Geometry: final body of the model. Coordinates: model frame, mm. A direction names the side the tool comes from. Give positions to 0.01 mm unless a question says otherwise; leave off trailing zeros. Loops run counter-clockwise (first coordinate to the right, second up) from the corner with the lowest first, then second, coordinate; pieces in that order, holes last. Notation, with made-up numbers: (-7.5, -10) -> (-2.5, -10) arc R13 ccw to (-2.5, 1) -> close; hole circle Ø5 at (1.5, -32.75). An arc over 180 degrees is marked (long way). One line per question, with ' | ' between items. Start each with the question number.
Item 1: Mould query, pull axis Z, two halves, no side actions, for faces 3 (the cylindrical face through (-1.521, 5.406, -5.712)), 4 (the cylindrical face through (-1.479, 19.248, -0.713)), 5 (the flat face through (0, 10, -11)). Classes: released by +Z, released by -Z, zero draft, split by the parting line, or undercut.
Item 2: Pin query (flat end, axial travel): P1, Ø9, axis at x = 9, z = -0.5, coming from the +Y side; P2, Ø9.5, axis at x = 12.5, y = 7, coming from the -Z side; P3, Ø3.5, axis at y = 15, z = -7, coming from the +X side. Return the tip coordinate at first contact, or that it passes through.
Item 3: Set-up query: faces 1 (the flat face through (-2, 20, -10)), 2 (the flat face through (11, 7, 0)). Return all of +Z, -Z, +X, -X, +Y, -Y with unobstructed straight access to the full face (end or side cutting, diameter ignored); none if empty.
Item 4: Section B-B on z = -7. Return loops of the section in (x, y).
Item 5: Section A-A on y = 5. Return loops of the section in (x, z).
Item 6: Section C-C on z = -10.75. Return loops of the section in (x, y).
Item 7: Material intervals for line 1 along Y through (x, z) = (-1, -7); line 2 along X through (y, z) = (9.5, -5.25); line 3 along Z through (x, y) = (7, 13.5), sorted ascending. Write a range as [from, to].
Item 8: Section D-D on x = 10. Return loops of the section in (y, z), then the cut area to 3 significant figures.
from build123d import *

# Parameters (mm, degrees)
BOSS_EXTRUDE1_DEPTH            = 20
F_2_7_2_7_DIAMETER_HOLE1_D     = 2.7
F_2_7_2_7_DIAMETER_HOLE1_DEPTH = 15
F_2_7_2_7_DIAMETER_HOLE1_TIP   = 0.811161836
SKETCH4_W                      = 20
SKETCH4_H                      = 3
CUT_EXTRUDE1_DEPTH             = 5
FILLET2_R                      = 2.5
FILLET3_R                      = 5


with BuildPart() as part:
    # Sketch1 → Boss-Extrude1 (new body)
    with BuildSketch(Plane(origin=(0, 0, 0), x_dir=(1, 0, 0), z_dir=(0, 1, 0))):
        Polygon((0, 0), (0, 17), (-3, 17), (-3, -3), (17, -3), (17, 0), align=None)
    extrude(amount=BOSS_EXTRUDE1_DEPTH)

    # Ø2.7 (2.7) Diameter Hole1
    with Locations(Plane(origin=(0, 0, 0), x_dir=(0, 0, -1), z_dir=(1, 0, 0))):
        with Locations((7, 5), (7, 15)):
            Hole(F_2_7_2_7_DIAMETER_HOLE1_D / 2, depth=F_2_7_2_7_DIAMETER_HOLE1_DEPTH)
            with Locations((0, 0, -(F_2_7_2_7_DIAMETER_HOLE1_DEPTH + F_2_7_2_7_DIAMETER_HOLE1_TIP / 2))):  # 118° drill point
                Cone(0, F_2_7_2_7_DIAMETER_HOLE1_D / 2, F_2_7_2_7_DIAMETER_HOLE1_TIP, mode=Mode.SUBTRACT)

    # Sketch4 → Cut-Extrude1 (cut)
    with BuildSketch(Plane(origin=(0, 20, 0), x_dir=(1, 0, 0), z_dir=(0, 1, 0))):
        with Locations((7, -1.5)):
            Rectangle(SKETCH4_W, SKETCH4_H)
    extrude(amount=-CUT_EXTRUDE1_DEPTH, mode=Mode.SUBTRACT)

    # Fillet2
    fillet2_edges = [part.edges().sort_by_distance(p)[0] for p in [
        (-1.5, 15, 0),
    ]]
    fillet(fillet2_edges, radius=FILLET2_R)
    fillet2_2_edges = [part.edges().sort_by_distance(p)[0] for p in [
        (-1.5, 20, 0),
    ]]
    fillet(fillet2_2_edges, radius=FILLET2_R - 0.0001)  # a hair under: the kernel refuses the full size

    # Fillet3
    fillet3_edges = [part.edges().sort_by_distance(p)[0] for p in [
        (0, 7.5, 0),
    ]]
    fillet(fillet3_edges, radius=FILLET3_R)


solid = part.part
Result sheet:
1) face 3: undercut | face 4: released by +Z | face 5: zero draft
2) P1: stops at y = 15 | P2: stops at z = 0 | P3: stops at x = 0
3) face 1: +Z, -Z, +X, -X, +Y | face 2: -Z, +X, +Y, -Y
4) outline: (-3, 0) -> (0, 0) -> (0, 3.65) -> (-3, 3.65) -> close; (-3, 6.35) -> (0, 6.35) -> (0, 13.65) -> (-3, 13.65) -> close; (-3, 16.35) -> (0, 16.35) -> (0, 20) -> (-3, 20) -> close
5) outline: (-3, -17) -> (0, -17) -> (0, -8.35) -> (-3, -8.35) -> close; (-3, -5.65) -> (0, -5.65) -> (0, -5) arc R5 cw to (5, 0) -> (17, 0) -> (17, 3) -> (-3, 3) -> close
6) outline: (-3, 0) -> (0, 0) -> (0, 20) -> (-3, 20) -> close
7) line 1: y = [0, 3.65], [6.35, 13.65], [16.35, 20] | line 2: x = [-3, 0] | line 3: z = [0, 3]
8) outline: (0, 0) -> (15, 0) -> (15, 3) -> (0, 3) -> close | area: 45.0 mm²
